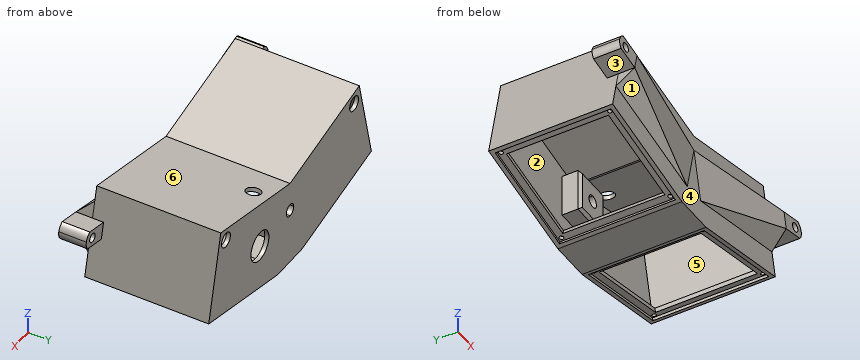
from build123d import *

# Parameters (mm, degrees)
EXTERNAL_DIMENSIONS_DEPTH             = 45
INTERNAL_CAVITY_DEPTH                 = 42
SKETCH5_W                             = 80.200000486
SKETCH5_H                             = 84.000000972
FIRST_CUTOUT_DEPTH                    = 2
SKETCH6_R                             = 1.5
SKETCH6_W                             = 70.200000486
SKETCH6_H                             = 74.000000972
SECOND_CUTOUT_HOLES_FOR_INSERTS_DEPTH = 3.1
SKETCH8_W                             = 29.263844186
SKETCH8_H                             = 31.126435476
TOPATTACHMENTSUPPORT_DEPTH            = 15
TOPATTACHMENT_SIZE                    = 2
TOP_HOLE_DEPTH                        = 20
BOTTOMSUPPORT_DEPTH                   = 12
CHAMFER1_SIZE                         = 12
LEFTCUT_DEPTH                         = 60
EXTRACUT_DEPTH                        = 100
SKETCH18_W                            = 12
SKETCH18_H                            = 20
BOTTOMATTACHMENT_DEPTH                = 20
BOTTOM_ATTACHMENT_ROUNDING_REACH      = 154.026
SKETCH19_R                            = 3.25
SKETCH20_R                            = 5.375
WIREEXIT_DEPTH                        = 10
SKETCH23_R                            = 5.375
CHARGERPORT_DEPTH                     = 10
SKETCH29_R                            = 10.9
CUT_EXTRUDE1_DEPTH                    = 10


with BuildPart() as part:
    # Sketch1 → External Dimensions (new, symmetric)
    with BuildSketch(Plane(origin=(0, 0, 0), x_dir=(1, 0, 0), z_dir=(0, 1, 0))):
        Polygon((0, 0), (83.973745957, -19.464069204), (98.60566805, 43.662366272), (14.631922093, 63.126435476), (-14.631922093, 63.126435476), (-98.60566805, 43.662366272), (-83.973745957, -19.464069204), align=None)
    extrude(amount=EXTERNAL_DIMENSIONS_DEPTH, both=True)

    # Sketch4 → Internal Cavity (cut, symmetric)
    with BuildSketch(Plane(origin=(0, 0, 0), x_dir=(1, 0, 0), z_dir=(0, 1, 0))):
        Polygon((-0.677403801, 2.922520161), (0.677403801, 2.922520161), (81.728629596, -15.864145243), (94.554142028, 39.468903028), (13.502915759, 58.255568541), (-13.502915759, 58.255568541), (-94.554142028, 39.468903028), (-81.728629596, -15.864145243), align=None)
    extrude(amount=INTERNAL_CAVITY_DEPTH, both=True, mode=Mode.SUBTRACT)

    # Sketch5 → First Cutout (cut)
    with BuildSketch(Plane(origin=(14.631922093, 0, -63.126435476), x_dir=(-0.9741733869698493, 0, -0.22580126686910412), z_dir=(0.22580126686910412, 0, -0.9741733869698493))):
        with Locations((-43.100000243, 0)):
            Rectangle(SKETCH5_W, SKETCH5_H)
    first_cutout = extrude(amount=-FIRST_CUTOUT_DEPTH, mode=Mode.SUBTRACT)

    # Sketch6 → Second Cutout + Holes for Inserts (cut)
    with BuildSketch(Plane(origin=(14.180319559, 0, -61.178088702), x_dir=(-0.9741733869698493, 0, -0.2258012668691041), z_dir=(0.2258012668691041, 0, -0.9741733869698493))):
        with Locations((-80.700000486, 39.500000486)):
            Circle(SKETCH6_R)
        with Locations((-5.499999514, 39.500000486)):
            Circle(SKETCH6_R)
        with Locations((-5.499999514, -39.500000486)):
            Circle(SKETCH6_R)
        with Locations((-80.700000486, -39.500000486)):
            Circle(SKETCH6_R)
        with Locations((-43.100000243, 0)):
            Rectangle(SKETCH6_W, SKETCH6_H)
    second_cutout_holes_for_inserts = extrude(amount=-SECOND_CUTOUT_HOLES_FOR_INSERTS_DEPTH, mode=Mode.SUBTRACT)

    # Mirror1: First Cutout, Second Cutout + Holes for Inserts across plane
    add(first_cutout.mirror(Plane(origin=(0, 0, 0), x_dir=(0, 0, 1), z_dir=(1, 0, 0))), mode=Mode.SUBTRACT)
    add(second_cutout_holes_for_inserts.mirror(Plane(origin=(0, 0, 0), x_dir=(0, 0, 1), z_dir=(1, 0, 0))), mode=Mode.SUBTRACT)

    # Sketch8 → TopAttachmentSupport (add)
    with BuildSketch(Plane(origin=(0, 43.5, 0), x_dir=(1, 0, 0), z_dir=(0, 1, 0))):
        with Locations((0, 21.563217738)):
            Rectangle(SKETCH8_W, SKETCH8_H)
    extrude(amount=-TOPATTACHMENTSUPPORT_DEPTH)

    # TopAttachment
    topattachment_edges = [part.edges().sort_by_distance(p)[0] for p in [
        (0, 28.5, -6),
        (0, 28.5, -37.126435476),
        (14.631922093, 28.5, -21.563217738),
        (-14.631922093, 28.5, -21.563217738),
    ]]
    chamfer(topattachment_edges, length=TOPATTACHMENT_SIZE)

    # Sketch9 → Top Hole (cut)
    with BuildSketch(Plane(origin=(0, 28.5, 0), x_dir=(-1, 0, 0), z_dir=(0, -1, 0))):
        with BuildLine():
            ThreePointArc((4.5, 21.563217738), (3.181980515, 24.745198253), (0, 26.063217738))
            Line((0, 26.063217738), (0, 17.063217738))
            ThreePointArc((0, 17.063217738), (3.181980515, 18.381237222), (4.5, 21.563217738))
        make_face()
        with BuildLine():
            Line((0, 17.063217738), (0, 26.063217738))
            ThreePointArc((0, 26.063217738), (-4.5, 21.563217738), (0, 17.063217738))
        make_face()
    extrude(amount=-TOP_HOLE_DEPTH, mode=Mode.SUBTRACT)

    # Sketch10 → BottomSupport (add)
    with BuildSketch(Plane.XZ.offset(45)):
        Polygon((-89.175695767, -2.978679395), (0, -23.648495823), (89.175695767, -2.978679395), (91.88531097, -14.668760038), (0, -35.966631548), (-91.88531097, -14.668760038), align=None)
    extrude(amount=BOTTOMSUPPORT_DEPTH)

    # Chamfer1
    chamfer1_edges = [part.edges().sort_by_distance(p)[0] for p in [
        (45.942655485, -45, -25.317695793),
        (44.587847884, -45, -13.313587609),
        (-44.587847884, -45, -13.313587609),
        (-45.942655485, -45, -25.317695793),
    ]]
    chamfer(chamfer1_edges, length=CHAMFER1_SIZE - 0.0001)  # a hair under: the kernel refuses the full size

    # Sketch14 → LeftCut (cut)
    with BuildSketch(Plane(origin=(0, 0, 0), x_dir=(0.9741733869698491, 0, -0.22580126686910457), z_dir=(0.22580126686910457, 0, 0.9741733869698491))):
        Polygon((2.558409664, -45), (-86.2, -57), (5.339860316, -57), align=None)
    leftcut = extrude(amount=-LEFTCUT_DEPTH, mode=Mode.SUBTRACT)

    # Mirror2: LeftCut across plane
    add(leftcut.mirror(Plane(origin=(0, 0, 0), x_dir=(0, 0, 1), z_dir=(1, 0, 0))), mode=Mode.SUBTRACT)

    # Sketch17 → ExtraCut (cut)
    with BuildSketch(Plane.XZ.offset(45)):
        Polygon((0, -11.330360098), (8.128845607, -46.400602029), (0, -48.284767272), (-8.128845607, -46.400602029), align=None)
    extrude(amount=EXTRACUT_DEPTH, mode=Mode.SUBTRACT)

    # Sketch18 → BottomAttachment (add)
    with BuildSketch(Plane(origin=(83.973745957, 0, 19.464069204), x_dir=(0.22580126686910407, 0, -0.9741733869698493), z_dir=(0.9741733869698493, 0, 0.22580126686910407))):
        with Locations((29.037735273, -47)):
            Rectangle(SKETCH18_W, SKETCH18_H)
    bottomattachment = extrude(amount=BOTTOMATTACHMENT_DEPTH)

    # Sketch19 → Bottom Attachment Rounding (cut, up to next)
    with BuildSketch(Plane(origin=(0, -37, 0), x_dir=(1, 0, 0), z_dir=(0, 1, 0)), mode=Mode.PRIVATE) as bottom_attachment_rounding_sk1:
        with Locations(Location((102.707670706, 6.001203881, 0), (0, 0, 270))):
            Circle(SKETCH19_R)
    bottom_attachment_rounding_tool1 = extrude(bottom_attachment_rounding_sk1.sketch, amount=-BOTTOM_ATTACHMENT_ROUNDING_REACH, mode=Mode.PRIVATE) & part.part
    # Sketch19 → Bottom Attachment Rounding (cut, up to next)
    with BuildSketch(Plane(origin=(0, -37, 0), x_dir=(1, 0, 0), z_dir=(0, 1, 0)), mode=Mode.PRIVATE) as bottom_attachment_rounding_sk2:
        with BuildLine():
            ThreePointArc((110.013971108, 4.307694379), (109.999984924, 7.753959807), (108.446258548, 10.830138501))
            Line((108.446258548, 10.830138501), (111.368778709, 10.152734701))
            Line((111.368778709, 10.152734701), (110.013971108, 4.307694379))
        make_face()
    bottom_attachment_rounding_tool2 = extrude(bottom_attachment_rounding_sk2.sketch, amount=-BOTTOM_ATTACHMENT_ROUNDING_REACH, mode=Mode.PRIVATE) & part.part
    # Sketch19 → Bottom Attachment Rounding (cut, up to next)
    with BuildSketch(Plane(origin=(0, -37, 0), x_dir=(1, 0, 0), z_dir=(0, 1, 0)), mode=Mode.PRIVATE) as bottom_attachment_rounding_sk3:
        with BuildLine():
            Line((110.013971108, 4.307694379), (108.659163507, -1.537345943))
            Line((108.659163507, -1.537345943), (105.736643346, -0.859942142))
            ThreePointArc((105.736643346, -0.859942142), (108.485263978, 1.219006062), (110.013971108, 4.307694379))
        make_face()
    bottom_attachment_rounding_tool3 = extrude(bottom_attachment_rounding_sk3.sketch, amount=-BOTTOM_ATTACHMENT_ROUNDING_REACH, mode=Mode.PRIVATE) & part.part
    bottom_attachment_rounding_1 = bottom_attachment_rounding_tool1.solids().sort_by_distance((102.707671, -37, -6.001204))[0]
    add(bottom_attachment_rounding_1, mode=Mode.SUBTRACT)
    bottom_attachment_rounding_2 = bottom_attachment_rounding_tool2.solids().sort_by_distance((110.209545, -37, -8.949999))[0]
    add(bottom_attachment_rounding_2, mode=Mode.SUBTRACT)
    bottom_attachment_rounding_3 = bottom_attachment_rounding_tool3.solids().sort_by_distance((108.14727, -37, -0.052736))[0]
    add(bottom_attachment_rounding_3, mode=Mode.SUBTRACT)
    bottom_attachment_rounding = bottom_attachment_rounding_1 + bottom_attachment_rounding_2 + bottom_attachment_rounding_3  # Bottom Attachment Rounding as one shape, for the pattern or mirror that repeats it

    # Mirror3: BottomAttachment, Bottom Attachment Rounding across plane
    add(bottomattachment.mirror(Plane(origin=(0, 0, 0), x_dir=(0, 0, 1), z_dir=(1, 0, 0))))
    add(bottom_attachment_rounding.mirror(Plane(origin=(0, 0, 0), x_dir=(0, 0, 1), z_dir=(1, 0, 0))), mode=Mode.SUBTRACT)

    # Sketch20 → WireExit (cut)
    with BuildSketch(Plane(origin=(40.135943543, 45, 9.303012195), x_dir=(0.22580126686910407, 0, -0.9741733869698493), z_dir=(0, -1, 0))):
        with Locations(Location((8.375, 36.625, 0), (0, 0, 180))):
            Circle(SKETCH20_R)
    wireexit = extrude(amount=WIREEXIT_DEPTH, mode=Mode.SUBTRACT)

    # Mirror4: WireExit across plane
    add(wireexit.mirror(Plane(origin=(0, 0, 0), x_dir=(0, 0, 1), z_dir=(1, 0, 0))), mode=Mode.SUBTRACT)

    # Sketch23 → ChargerPort (cut)
    with BuildSketch(Plane(origin=(0, 0, 0), x_dir=(0.9741733869698492, 0, 0.22580126686910437), z_dir=(-0.22580126686910437, 0, 0.9741733869698492))):
        with Locations((25, 33)):
            Circle(SKETCH23_R)
    extrude(amount=-CHARGERPORT_DEPTH, mode=Mode.SUBTRACT)

    # Sketch29 → Cut-Extrude1 (cut)
    with BuildSketch(Plane(origin=(0, 45, 0), x_dir=(1, 0, 0), z_dir=(0, 1, 0))):
        with Locations(Location((36.541162656, 24.789179732, 0), (0, 0, 270))):
            Circle(SKETCH29_R)
    extrude(amount=-CUT_EXTRUDE1_DEPTH, mode=Mode.SUBTRACT)


solid = part.part
The listing builds one solid part. Answer for the finished solid, in the listing's coordinates (mm). Face numbers are marked on the shaded views. A direction names the side the tool comes from. Give positions to 0.01 mm unless a question says otherwise; leave off trailing zeros. Loops run counter-clockwise (first coordinate to the right, second up) from the corner with the lowest first, then second, coordinate; pieces in that order, holes last. Notation, with made-up numbers: (61.25, 85) - (104.25, 85) arc R28 cw to (104.25, 106) - close; hole circle Ø1 at (-38, 85). An arc over 180 degrees is marked (long way). Answer as a JSON object with one key per item and string values.
1. Flat-ended cylindrical pins translate along their axes: pin 1 Ø6 at (x, z) = (81, 13.5) entering from -Y; pin 2 Ø6 at (x, y) = (19.5, 33) entering from -Z; pin 3 Ø19.5 at (x, z) = (36.54, -24.79) entering from -Y; pin 4 Ø16 at (x, z) = (-69, -52) entering from +Y. Find the tip coordinate at first contact, or state that the pin passes through.
Determined:
{"pin 1": "y = -45", "pin 2": "z = -62.69", "pin 3": "y = -50.72", "pin 4": "y = 45"}
2. For a pull along Y with two mould halves and no side action, classify the marked faces 1, 2 and 3 as pulls with the +Y half, pulls with the -Y half, needs draft (parallel to the pull), parting line crosses it, or undercut.
Determined:
{"face 1": "pulls with the -Y half", "face 2": "undercut", "face 3": "needs draft"}
3. A cutting plane is placed at C-C (x = -79). Write down the section's boundary in (y, z).
Determined:
{"outline": "(-55.63, -3.93) - (-55.15, -19.55) - (-45, -29.97) - (-45, -48.21) - (-42, -48.21) - (-42, -46.15) - (-37, -46.15) - (-37, -43.07) - (-42, -43.07) - (-42, 15.23) - (42, 15.23) - (42, 14.63) - (45, 14.63) - (45, 18.31) - (-45, 18.31) - (-45, 6.98) - close; (37, -46.15) - (42, -46.15) - (42, -48.21) - (45, -48.21) - (45, 4.2) - (42, 4.2) - (42, -43.07) - (37, -43.07) - close"}
4. For the marked faces 4, 5 and 6, determine the directions among +Z, -Z, +X, -X, +Y, -Y from which every point of the face is accessible in a straight line to the end or side of a thin tool.
Determined:
{"face 4": "-Z, -Y", "face 5": "none", "face 6": "+Z, +Y, -Y"}
5. A cutting plane is placed at B-B (z = -51.5). Write down the section's boundary in (x, y).
Determined:
{"outline": "(-64.79, -45) - (64.79, -45) - (64.79, -42) - (55.93, -42) - (55.93, -37) - (42.65, -37) - (42.65, -42) - (-42.65, -42) - (-42.65, -37) - (-55.93, -37) - (-55.93, -42) - (-64.79, -42) - close; (-64.79, 42) - (-55.93, 42) - (-55.93, 37) - (-42.65, 37) - (-42.65, 42) - (42.65, 42) - (42.65, 37) - (55.93, 37) - (55.93, 42) - (64.79, 42) - (64.79, 45) - (-64.79, 45) - close"}
6. Find the intervals of material crossed by L1, parallel to Y at x = 2, z = -48; L2, parallel to X at y = 33.5, z = -7.5; L3, parallel to Y at x = -98, z = -7.5, in increasing order. Write a range as [from, to].
Determined:
{"L1": "[-45, -42], [42, 45]", "L2": "[-90.22, -87.14], [-14.63, 14.63], [87.14, 90.22]", "L3": "[-57, -37]"}
7. A cutting plane is placed at D-D (x = -46.5). Write down the section's boundary in (y, z).
Determined:
{"outline": "(-51.26, -6.98) - (-50.5, -31.86) - (-45, -37.51) - (-45, -55.74) - (-42, -55.74) - (-42, -53.69) - (-37, -53.69) - (-37, -50.61) - (-42, -50.61) - (-42, 7.7) - (42, 7.7) - (42, -50.61) - (37, -50.61) - (37, -53.69) - (42, -53.69) - (42, -55.74) - (45, -55.74) - (45, 10.78) - (-45, 10.78) - (-45, -0.55) - close"}
